```python
from build123d import *

# Parameters (mm, degrees)
F0_R     = 41.275
F1_DEPTH = 3.175
F2_R     = 38.2337964231
F2_R_2   = 36.8557965157
F3_DEPTH = 0.79375
F5_DEPTH = 0.79375


# Not quite as in the source:
# - a length typed as a fraction of an inch, garbled in the dataset ("3 / 203.2 mm" for 3/8 in), is restored


with BuildPart() as f1:
    # F0 (on Top) → F1 (new body)
    with BuildSketch(Plane.XY):
        Circle(F0_R)
    extrude(amount=F1_DEPTH)

    # F2 (on face) → F3 (cut)
    with BuildSketch(Plane.XY.offset(3.175)):
        Circle(F2_R)
        Circle(F2_R_2, mode=Mode.SUBTRACT)
    extrude(amount=-F3_DEPTH, mode=Mode.SUBTRACT)

    # F4 (on face) → F5 (cut)
    with BuildSketch(Plane.XY.offset(3.175)):
        Polygon((25.4, 0), (0, 25.4), (-25.4, 25.4), (-25.4, 0), (0, -25.4), (25.4, -25.4), align=None)
    extrude(amount=-F5_DEPTH, mode=Mode.SUBTRACT)


solid = f1.part
```
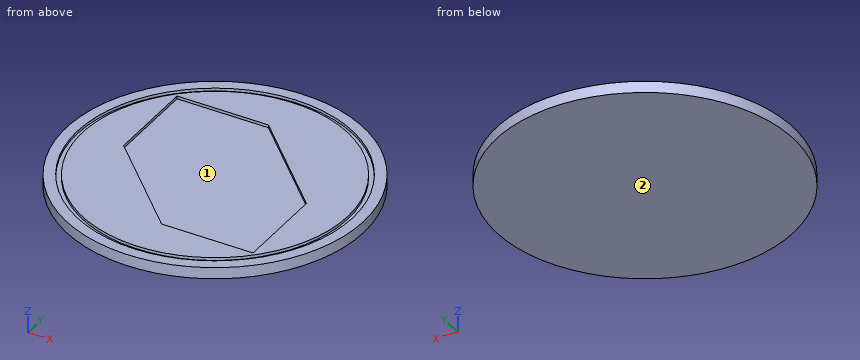
Here's how the part is built. I have some questions about the finished solid (model axes, mm). Face numbers are marked on the shaded views. Coordinates: 2 decimals unless noted, no trailing zeros. Loops run counter-clockwise (first coordinate to the right, second up) from the corner with the lowest first, then second, coordinate; pieces in that order, holes last. Notation, with made-up numbers: (53.5, 21.25) - (72.5, 21.25) arc R35 ccw to (72.5, 55.25) - close; hole circle Ø9 at (33.5, -5). An arc over 180 degrees is marked (long way). Return JSON: item names as keys, results as strings. Group by question number.
Item 1: If we section it at B-B on x = 17: Write out the boundary of the cut face in (y, z) (1 decimal).
Item 2: If we section it at D-D on y = -28: Write out the boundary of the cut face in (x, z) (3 decimals), and give its area (3 significant figures).
Item 3: We'd pull the mould along X, two halves only. Please class the marked faces 1 and 2: +X half, -X half, draft (parallel to the pull), parting line (faces both ways), or undercut.
Item 4: If we section it at C-C on z = 1.55: Write out the boundary of the cut face in (x, y) (3 decimals).
Item 5: I need wall thicknesses on line 1 (Y direction, x = 0, z = 2.9) (3 decimals); line 2 (Z direction, x = -2, y = -37); line 3 (X direction, y = -15.5, z = 2.5). Which ranges of each line are inside material? Lowest first, please. Write a range as from..to.
Item 6: Will these pins go through, and if not, where does the flat tip stop? P1, Ø15, axis at x = -3.5, y = -9, coming from the +Z side; P2, Ø0.6, axis at y = 15, z = 3, coming from the +X side; P3, Ø0.9, axis at x = -16, z = 3, coming from the -Y side.
Item 7: If we section it at A-A on y = 34: Write out the boundary of the cut face in (x, z) (3 decimals), and give its area (3 significant figures).
Calculated:
{
 "1": {"outline": "(-37.6, 0) - (37.6, 0) - (37.6, 3.2) - (34.2, 3.2) - (34.2, 2.4) - (32.7, 2.4) - (32.7, 3.2) - (8.4, 3.2) - (8.4, 2.4) - (-25.4, 2.4) - (-25.4, 3.2) - (-32.7, 3.2) - (-32.7, 2.4) - (-34.2, 2.4) - (-34.2, 3.2) - (-37.6, 3.2) - close"},
 "2": {"outline": "(-30.325, 0) - (30.325, 0) - (30.325, 3.175) - (26.035, 3.175) - (26.035, 2.381) - (23.966, 2.381) - (23.966, 3.175) - (-23.966, 3.175) - (-23.966, 2.381) - (-26.035, 2.381) - (-26.035, 3.175) - (-30.325, 3.175) - close", "area": "189 mm^2"},
 "3": {"face 1": "undercut", "face 2": "draft"},
 "4": {"outline": "circle Ø82.55 at (0, 0)"},
 "5": {"line 1": "y = -41.275..-38.234, -36.856..-25.4, 25.4..36.856, 38.234..41.275", "line 2": "z = 0..2.38", "line 3": "x = -38.25..-34.95, -33.44..-9.9, 25.4..33.44, 34.95..38.25"},
 "6": {"P1": "stops at z = 2.38", "P2": "stops at x = 38.57", "P3": "stops at y = -38.23"},
 "7": {"outline": "(-23.401, 0) - (23.401, 0) - (23.401, 3.175) - (17.488, 3.175) - (17.488, 2.381) - (14.225, 2.381) - (14.225, 3.175) - (-14.225, 3.175) - (-14.225, 2.381) - (-17.488, 2.381) - (-17.488, 3.175) - (-23.401, 3.175) - close", "area": "143 mm^2"}
}
